Geometry check sheet. Reference: the model listing, model coordinates, mm. A direction names the side the tool comes from. Round coordinates to 2 decimals unless told otherwise and drop trailing zeros. Order: outer loops, then holes, each group sorted by start corner. A loop starts at its lowest first (then second) coordinate and runs counter-clockwise, first axis right, second up.
(1) Go/stop test with flat-tipped pins: pin 1 (2 mm diameter, centred on y = 5, z = -8.5, fed in from -X); pin 2 (1 mm diameter, centred on x = -10, y = 2, fed in from -Z); pin 3 (2 mm diameter, centred on x = -2, z = -3, fed in from -Y); pin 4 (3 mm diameter, centred on x = -0.5, z = -6, fed in from -Y). Record where each tip stops, or that it passes through.
(2) Sectioned sample at A-A (x = 0). Record the boundary of the cut face in (y, z), plus the area to 3 significant figures.
(3) Sectioned sample at C-C (y = -7.75). Record the boundary of the cut face in (x, z), plus the area to 3 significant figures.
(4) Material ranges on line 1 along Y through (x, z) = (1.25, -11.5) (3 decimals); line 2 along X through (y, z) = (6.5, -8); line 3 along X through (y, z) = (-5.25, -5.5), recorded low to high.
(5) Release check for a two-part mould opening along Y. For faces 1 (the face through (0, 7.65, -10)), 2 (the face through (-0.215, 2.71, -9.798)), 3 (the face through (-1, 2, -10)), 4 (the face through (-0.2, 3.7, -10.1)) record: +Y half, -Y half, draft (parallel to the pull), parting line (faces both ways), or undercut.
(6) Sectioned sample at B-B (y = 4.5). Record the boundary of the cut face in (x, z).
(7) Set-up check for faces 5 (the face through (-0.215, 7.157, -9.798)), 6 (the face through (-0.303, 3.771, -13.797)), 7 (the face through (-0.1, -10.2, -6.8)), 8 (the face through (-1, 6.65, -10)): record each of +Z, -Z, +X, -X, +Y, -Y from which the full face is reachable in a straight line by a thin tool's end or side.
from build123d import *

# Parameters (mm, degrees)
F1_ANGLE    = 180
F2_T4_ANGLE = 248.1806251609
F2_S5_R     = 11.8
F2_T6_DEPTH = 17
F3_T4_ANGLE = 247.7679532438
F3_S5_R     = 11.8
F3_T6_DEPTH = 17


# Not quite as in the source:
# - a fillet or chamfer that OpenCascade refuses, or shapes differently, is made with other operations: its cross-section is extruded or revolved along the edge and cut away or added


with BuildPart() as f1:
    # F0 (on Top) → F1 (revolve)
    with BuildSketch(Plane.XY):
        Polygon((-11.8, 5.65), (-11.8, 6.65), (-13.8, 6.65), (-13.8, 0), (-7.8, -10.95), (-6.8, -10.95), (-6.8, -9.45), (-4.8, -9.45), (-4.8, -7.45), (-9.8, 1), (-11.8, 1), (-11.8, 2), (-9.8, 2), (-9.8, 5.65), align=None)
        Polygon((-13.8, 6.65), (-11.8, 6.65), (-9.8, 6.65), (-9.8, 7.65), (-13.8, 7.65), align=None)
    revolve(axis=Axis((0, 0, 0), (0, -1, 0)), revolution_arc=F1_ANGLE)

    # F2: chamfer of 2.25 on 1 edges, made by hand


with BuildPart() as f2_tool2:
    # F2_s3 → F2_t4 (revolve)
    with BuildSketch(Plane(origin=(0, 0, 0), x_dir=(0, 1, 0), z_dir=(0.5604989803, 0, 0.8281551142))):
        Polygon((-0.9364000214, 8.6542011708), (1, 12.05), (1, 9.8), align=None)
    revolve(axis=Axis((0, 1, 0), (0, -1, 0)), revolution_arc=F2_T4_ANGLE)

    # F2_s5 → F2_t6 (intersect, symmetric)
    with BuildSketch(Plane.XZ):
        Circle(F2_S5_R)
    extrude(amount=F2_T6_DEPTH, both=True, mode=Mode.INTERSECT)


with BuildPart() as f1_1:
    add(f1.part)

    # F2_t1: cut F2_tool2
    add(f2_tool2.part, mode=Mode.SUBTRACT)

    # F3: chamfer of 2.25 on 1 edges, made by hand


with BuildPart() as f3_tool2:
    # F3_s3 → F3_t4 (revolve)
    with BuildSketch(Plane(origin=(0, 0, 0), x_dir=(0, 1, 0), z_dir=(0.5575129654, 0, 0.830168232))):
        Polygon((5.65, 12.05), (3.4, 9.8), (5.65, 9.8), align=None)
    revolve(axis=Axis((0, 5.65, 0), (0, -1, 0)), revolution_arc=F3_T4_ANGLE)

    # F3_s5 → F3_t6 (intersect, symmetric)
    with BuildSketch(Plane.XZ.offset(-4.5)):
        Circle(F3_S5_R)
    extrude(amount=F3_T6_DEPTH, both=True, mode=Mode.INTERSECT)


with BuildPart() as f1_2:
    add(f1_1.part)

    # F3_t1: cut F3_tool2
    add(f3_tool2.part, mode=Mode.SUBTRACT)


solid = f1_2.part
Answer below:
1. pin 1: stops at x = -11.58
1. pin 2: stops at z = -10.01
1. pin 3: passes through
1. pin 4: stops at y = -10.95
2. outline: (-10.95, -7.8) - (0, -13.8) - (7.65, -13.8) - (7.65, -9.8) - (6.65, -9.8) - (6.65, -11.8) - (5.4, -11.8) - (3.4, -9.8) - (2, -9.8) - (2, -11.8) - (0.86, -11.8) - (-0.94, -8.65) - (-7.45, -4.8) - (-9.45, -4.8) - (-9.45, -6.8) - (-10.95, -6.8) - close
2. area: 68.5 mm2
3. outline: (-9.55, 0) arc R9.55 ccw to (9.55, 0) - (4.8, 0) arc R4.8 cw to (-4.8, 0) - close
3. area: 107 mm2
4. line 1: y = -4.074 to 0.725, 2 to 5.168, 6.65 to 7.65
4. line 2: x = -11.24 to -8.67, 8.67 to 11.24
4. line 3: x = -9.44 to -2.64, 2.64 to 9.44
5. face 1: +Y half
5. face 2: draft
5. face 3: undercut
5. face 4: undercut
6. outline: (-13.8, 0) arc R13.8 ccw to (13.8, 0) - (10.9, 0) arc R10.9 cw to (-10.9, 0) - close
7. face 5: +Z, +Y
7. face 6: -Z, +Y, -Y
7. face 7: +Z, -Y
7. face 8: +Z
